Design review of the part built by this model. Coordinates are the model's own, in mm. Face numbers are marked on the shaded views. A direction names the side the tool comes from. Give positions to 0.01 mm unless a question says otherwise; leave off trailing zeros. Write each loop counter-clockwise with the first axis right and the second up, starting at its lowest first coordinate (ties: lowest second). Pieces come first, ordered by that corner, then holes.
```python
from build123d import *

# Parameters (mm, degrees)
BOSS_EXTRUDE1_DEPTH      = 10.1
BOSS_EXTRUDE1_DEPTH_BACK = 8.6
SKETCH1_R                = 1.55
BOSS_EXTRUDE2_DEPTH      = 8.7
SKETCH3_R                = 1.95
BOSS_EXTRUDE3_DEPTH      = 1.85
BOSS_EXTRUDE4_DEPTH      = 26
SKETCH5_W                = 5.1
SKETCH5_H                = 2.5
BOSS_EXTRUDE5_DEPTH      = 2.2
CHAMFER1_SIZE            = 1
CUT_EXTRUDE1_DEPTH       = 14.8
SKETCH7_W                = 3
SKETCH7_H                = 6.7
CUT_EXTRUDE2_DEPTH       = 1.5
FILLET1_R                = 2
SKETCH8_W                = 7.6
SKETCH8_H                = 8.5
BOSS_EXTRUDE6_DEPTH      = 1.5
SKETCH9_W                = 6.939646177
SKETCH9_H                = 7.5
CUT_EXTRUDE3_DEPTH       = 2
SKETCH10_W               = 3.7
SKETCH10_H               = 2
BOSS_EXTRUDE7_DEPTH      = 1
FILLET2_R                = 1.5
BOSS_EXTRUDE8_DEPTH      = 1
SKETCH12_R               = 1
BOSS_EXTRUDE9_DEPTH      = 1
SKETCH13_R               = 1.3
CUT_EXTRUDE4_DEPTH       = 8.7
SKETCH14_W               = 5
SKETCH14_H               = 5
SKETCH14_R               = 1.5
BOSS_EXTRUDE10_DEPTH     = 1.35
FILLET3_R                = 1


with BuildPart() as part:
    # Sketch1 → Boss-Extrude1 (new, two sides: drawn at the far end of the back side and taken through both)
    with BuildSketch(Plane.XY.offset(-BOSS_EXTRUDE1_DEPTH_BACK)):
        with BuildLine():
            Line((-11.175, -25.5), (11.175, -25.5))
            Line((11.175, -25.5), (11.175, 7.3))
            ThreePointArc((11.175, 7.3), (10.003427125, 10.128427125), (7.175, 11.3))
            Line((7.175, 11.3), (-7.175, 11.3))
            ThreePointArc((-7.175, 11.3), (-10.003427125, 10.128427125), (-11.175, 7.3))
            Line((-11.175, 7.3), (-11.175, -25.5))
        make_face()
        with Locations((-8.875, -20)):
            Circle(SKETCH1_R, mode=Mode.SUBTRACT)
        with Locations(Location((8.875, -20, 0), (0, 0, 180))):
            Circle(SKETCH1_R, mode=Mode.SUBTRACT)
    extrude(amount=BOSS_EXTRUDE1_DEPTH + BOSS_EXTRUDE1_DEPTH_BACK)

    # Sketch2 → Boss-Extrude2 (add)
    with BuildSketch(Plane.XY.offset(10.1)):
        with BuildLine():
            Line((-1.897366596, 1.85), (1.897366596, 1.85))
            ThreePointArc((1.897366596, 1.85), (2.65, 0), (1.897366596, -1.85))
            Line((1.897366596, -1.85), (-1.897366596, -1.85))
            ThreePointArc((-1.897366596, -1.85), (-2.65, 0), (-1.897366596, 1.85))
        make_face()
    extrude(amount=BOSS_EXTRUDE2_DEPTH)

    # Sketch3 → Boss-Extrude3 (add)
    with BuildSketch(Plane.XY.offset(10.1)):
        with Locations(Location((0, -11, 0), (0, 0, 180))):
            Circle(SKETCH3_R)
    extrude(amount=BOSS_EXTRUDE3_DEPTH)

    # Sketch4 → Boss-Extrude4 (add)
    with BuildSketch(Plane.XZ.offset(25.5)):
        with BuildLine():
            Line((-7.252758096, -8.6), (7.252758096, -8.6))
            ThreePointArc((7.252758096, -8.6), (9.911079132, -5.322876144), (11.175, -1.296871235))
            Line((11.175, -1.296871235), (11.175, 1.296871235))
            ThreePointArc((11.175, 1.296871235), (9.911079132, 5.322876144), (7.252758096, 8.6))
            Line((7.252758096, 8.6), (-7.252758096, 8.6))
            ThreePointArc((-7.252758096, 8.6), (-9.911079132, 5.322876144), (-11.175, 1.296871235))
            Line((-11.175, 1.296871235), (-11.175, -1.296871235))
            ThreePointArc((-11.175, -1.296871235), (-9.911079132, -5.322876144), (-7.252758096, -8.6))
        make_face()
    extrude(amount=BOSS_EXTRUDE4_DEPTH)

    # Sketch5 → Boss-Extrude5 (add)
    with BuildSketch(Plane(origin=(0, 0, -8.6), x_dir=(-1, 0, 0), z_dir=(0, 0, -1))):
        with Locations((0, -31.2)):
            Rectangle(SKETCH5_W, SKETCH5_H)
    boss_extrude5 = extrude(amount=BOSS_EXTRUDE5_DEPTH)

    # Mirror1: Boss-Extrude5 across plane
    add(boss_extrude5.mirror(Plane.XY))

    # Chamfer1
    chamfer1_edges = [part.edges().sort_by_distance(p)[0] for p in [
        (0, -32.45, 8.6),
        (0, -32.45, -8.6),
    ]]
    chamfer(chamfer1_edges, length=CHAMFER1_SIZE)

    # Sketch6 → Cut-Extrude1 (cut)
    with BuildSketch(Plane.XZ.offset(51.5)):
        with BuildLine():
            Line((-11.175, 3.35), (-9.315980893, 3.35))
            ThreePointArc((-9.315980893, 3.35), (-9.9, 0), (-9.315980893, -3.35))
            Line((-9.315980893, -3.35), (-11.175, -3.35))
            Line((-11.175, -3.35), (-11.175, 3.35))
        make_face()
        with BuildLine():
            Line((11.175, -3.35), (9.315980893, -3.35))
            ThreePointArc((9.315980893, -3.35), (9.9, 0), (9.315980893, 3.35))
            Line((9.315980893, 3.35), (11.175, 3.35))
            Line((11.175, 3.35), (11.175, -3.35))
        make_face()
    extrude(amount=-CUT_EXTRUDE1_DEPTH, mode=Mode.SUBTRACT)

    # Sketch7 → Cut-Extrude2 (cut)
    with BuildSketch(Plane.XZ.offset(51.5)):
        with Locations((-9.239646177, 0)):
            Rectangle(SKETCH7_W, SKETCH7_H)
        with Locations((9.239646177, 0)):
            Rectangle(SKETCH7_W, SKETCH7_H)
    extrude(amount=-CUT_EXTRUDE2_DEPTH, mode=Mode.SUBTRACT)

    # Fillet1
    fillet1_edges = [part.edges().sort_by_distance(p)[0] for p in [
        (9.9, -50, 0),
        (-9.9, -50, 0),
    ]]
    fillet(fillet1_edges, radius=FILLET1_R)

    # Sketch8 → Boss-Extrude6 (add)
    with BuildSketch(Plane(origin=(0, 0, -8.6), x_dir=(-1, 0, 0), z_dir=(0, 0, -1))):
        with Locations((0, -47.25)):
            Rectangle(SKETCH8_W, SKETCH8_H)
    extrude(amount=BOSS_EXTRUDE6_DEPTH)

    # Sketch9 → Cut-Extrude3 (cut)
    with BuildSketch(Plane(origin=(0, 0, -8.6), x_dir=(-1, 0, 0), z_dir=(0, 0, -1))):
        with Locations((7.269823089, -47.75)):
            Rectangle(SKETCH9_W, SKETCH9_H)
        with Locations((-7.269823089, -47.75)):
            Rectangle(SKETCH9_W, SKETCH9_H)
    extrude(amount=-CUT_EXTRUDE3_DEPTH, mode=Mode.SUBTRACT)

    # Sketch10 → Boss-Extrude7 (add)
    with BuildSketch(Plane(origin=(0, 0, -6.6), x_dir=(-1, 0, 0), z_dir=(0, 0, -1))):
        with Locations((-5.65, -47.5)):
            Rectangle(SKETCH10_W, SKETCH10_H)
        with Locations((5.65, -47.5)):
            Rectangle(SKETCH10_W, SKETCH10_H)
    extrude(amount=BOSS_EXTRUDE7_DEPTH)

    # Fillet2
    fillet2_edges = [part.edges().sort_by_distance(p)[0] for p in [
        (0, -51.5, -10.1),
    ]]
    fillet(fillet2_edges, radius=FILLET2_R)

    # Sketch11 → Boss-Extrude8 (add)
    with BuildSketch(Plane.XZ.offset(51.5)):
        with BuildLine():
            Line((-2.523885893, 4.2), (2.523885893, 4.2))
            ThreePointArc((2.523885893, 4.2), (0, -4.9), (-2.523885893, 4.2))
        make_face()
    extrude(amount=BOSS_EXTRUDE8_DEPTH)

    # Sketch12 → Boss-Extrude9 (add)
    with BuildSketch(Plane.XZ.offset(52.5)):
        with Locations(Location((0, 0, 0), (0, 0, 270))):
            Circle(SKETCH12_R)
    extrude(amount=BOSS_EXTRUDE9_DEPTH)

    # Sketch13 → Cut-Extrude4 (cut)
    with BuildSketch(Plane.XY.offset(18.8)):
        Circle(SKETCH13_R)
    extrude(amount=-CUT_EXTRUDE4_DEPTH, mode=Mode.SUBTRACT)

    # Sketch14 → Boss-Extrude10 (add, symmetric)
    with BuildSketch(Plane.XY):
        with Locations((0, 13.8)):
            Rectangle(SKETCH14_W, SKETCH14_H)
        with Locations(Location((0, 13.8, 0), (0, 0, 180))):
            Circle(SKETCH14_R, mode=Mode.SUBTRACT)
    extrude(amount=BOSS_EXTRUDE10_DEPTH, both=True)

    # Fillet3
    fillet3_edges = [part.edges().sort_by_distance(p)[0] for p in [
        (9.371354111, -51.5, 6.224164371),
        (-10.057256253, -51.5, -5.041239595),
        (0, -43, -10.1),
        (10.057256253, -51.5, -5.041239595),
        (2.5, 11.3, 0),
        (-2.5, 11.3, 0),
        (0, -51.5, 8.6),
        (-9.371354111, -51.5, 6.224164371),
    ]]
    fillet(fillet3_edges, radius=FILLET3_R)


solid = part.part
```
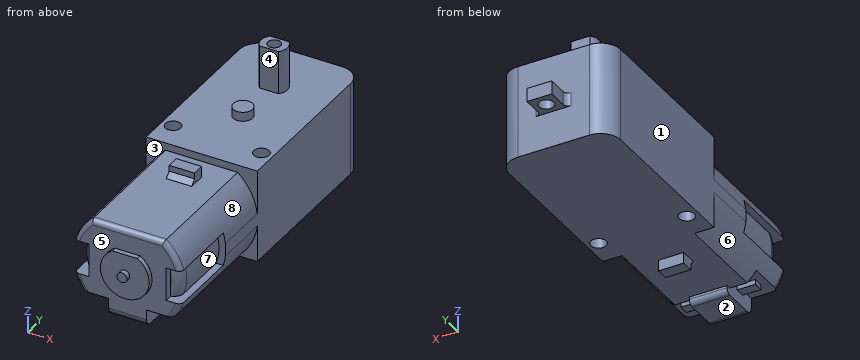
(1) Consider section B-B, the plane z = 14.25. Give the boundary of the cut face in (x, y).
Resolved:
outline: (-1.9, -1.85) - (1.9, -1.85) arc R2.65 ccw to (1.9, 1.85) - (-1.9, 1.85) arc R2.65 ccw to start; hole circle Ø2.6 at (0, 0)
(2) Consider section C-C, the plane x = -6. Give the boundary of the cut face in (y, z).
Resolved:
outline: (-51.5, -6.6) - (-48.5, -6.6) - (-48.5, -7.6) - (-46.5, -7.6) - (-46.5, -6.6) - (-44, -6.6) - (-44, -8.6) - (11.3, -8.6) - (11.3, 10.1) - (-25.5, 10.1) - (-25.5, 8.6) - (-50.5, 8.6) arc R1 ccw to (-51.5, 7.6) - close
(3) To check wall thickness, follow L1, parallel to X at y = 13.8, z = -0.3; L2, parallel to Y at x = 0, z = -0.4; L3, parallel to Y at x = 0, z = 14.5. State the ranges of each line that lie inside material, in increasing order.
Resolved:
L1: x = -2.5 to -1.5, 1.5 to 2.5
L2: y = -53.5 to 12.3, 15.3 to 16.3
L3: y = -1.85 to -1.3, 1.3 to 1.85
(4) Consider section D-D, the plane y = -11. Give the boundary of the cut face in (x, z) (3 decimals).
Resolved:
outline: (-11.175, -8.6) - (11.175, -8.6) - (11.175, 10.1) - (1.95, 10.1) - (1.95, 11.95) - (-1.95, 11.95) - (-1.95, 10.1) - (-11.175, 10.1) - close
(5) Clearance check with flat-ended pins moving along their axes: P1, Ø2, axis at x = 5, z = -6, coming from the +Y side; P2, Ø7, axis at x = 1, z = 4, coming from the +Y side; P3, Ø3, axis at y = -34.5, z = 5.5, coming from the -X side; P4, Ø3, axis at x = -9, z = -5, coming from the -Y side. State where each tip first meets the part, or that it passes through.
Resolved:
P1: stops at y = 11.3
P2: stops at y = 16.3
P3: stops at x = -10.51
P4: stops at y = -51.5
(6) Mouldability with a two-part tool opening along Z and no side actions: class the marked faces 6, 7 and 8 as pulls with the +Z half, pulls with the -Z half, needs draft (parallel to the pull), parting line crosses it, or undercut.
Resolved:
face 6: pulls with the -Z half
face 7: undercut
face 8: pulls with the +Z half
(7) Consider section A-A, the plane y = -20. Give the boundary of the cut face in (x, z) (3 decimals), then the cut area to 3 significant figures.
Resolved:
outline: (-11.175, -8.6) - (-10.425, -8.6) - (-10.425, 10.1) - (-11.175, 10.1) - close; (-7.325, -8.6) - (7.325, -8.6) - (7.325, 10.1) - (-7.325, 10.1) - close; (10.425, -8.6) - (11.175, -8.6) - (11.175, 10.1) - (10.425, 10.1) - close
area: 302 mm2
(8) Tool access review of the marked faces 1, 2, 3, 4 and 5: name each direction out of +Z, -Z, +X, -X, +Y, -Y from which nothing blocks a thin tool from reaching the whole face with its end or side.
Resolved:
face 1: +Z, -Z, -X, +Y, -Y
face 2: -Z, +X, -X, -Y
face 3: +Z
face 4: +Z, +X, -X
face 5: -Y
